```python
from build123d import *

# Parameters (mm, degrees)
SKETCH_1_R          = 5
EXTRUDE_4_DEPTH     = 12
FILLET_1_R          = 0.6
FILLET_2_R          = 0.6
EXTRUDE_5_DEPTH     = 6
SKETCH_3_R          = 2.55
CUT_EXTRUDE_1_DEPTH = 6
CHAMFER_1_SIZE      = 0.5
CHAMFER_4_SIZE      = 0.5
FILLET_4_R          = 0.5
FILLET_5_R          = 0.5
SKETCH_4_W          = 6.329239392
SKETCH_4_H          = 8
EXTRUDE_6_DEPTH     = 3.5
SKETCH_5_R          = 1.2
CUT_EXTRUDE_2_DEPTH = 3.5
FILLET_7_R          = 0.5


with BuildPart() as part:
    # ｽｹｯﾁ1 → ﾎﾞｽ - 押し出し4 (new body)
    with BuildSketch(Plane(origin=(0, 0, 0), x_dir=(1, 0, 0), z_dir=(0, 1, 0))):
        with Locations(Location((0, 0, 0), (0, 0, 270))):
            Circle(SKETCH_1_R)
        Polygon((-2.5, -0.925), (-2.5, 0.925), (-0.925, 0.925), (-0.925, 2.5), (0.925, 2.5), (0.925, 0.925), (2.5, 0.925), (2.5, -0.925), (0.925, -0.925), (0.925, -2.5), (-0.925, -2.5), (-0.925, -0.925), align=None, mode=Mode.SUBTRACT)
    extrude(amount=EXTRUDE_4_DEPTH)

    # ﾌｨﾚｯﾄ1
    fillet_1_edges = [part.edges().sort_by_distance(p)[0] for p in [
        (0.925, 6, -0.925),
    ]]
    fillet(fillet_1_edges, radius=FILLET_1_R)

    # ﾌｨﾚｯﾄ2
    fillet_2_edges = [part.edges().sort_by_distance(p)[0] for p in [
        (-0.925, 6, -0.925),
        (-0.925, 6, 0.925),
        (0.925, 6, 0.925),
    ]]
    fillet(fillet_2_edges, radius=FILLET_2_R)

    # ｽｹｯﾁ2 → ﾎﾞｽ - 押し出し5 (add)
    with BuildSketch(Plane.XZ):
        Polygon((6.92820323, 0), (3.464101615, 6), (-3.464101615, 6), (-6.92820323, 0), (-3.464101615, -6), (3.464101615, -6), align=None)
    extrude(amount=EXTRUDE_5_DEPTH)

    # ｽｹｯﾁ3 → ｶｯﾄ - 押し出し1 (cut)
    with BuildSketch(Plane.XZ.offset(6)):
        with Locations(Location((0, 0, 0), (0, 0, 270))):
            Circle(SKETCH_3_R)
    extrude(amount=-CUT_EXTRUDE_1_DEPTH, mode=Mode.SUBTRACT)

    # 面取り1
    chamfer_1_edges = [part.edges().sort_by_distance(p)[0] for p in [
        (0, -6, 2.55),
        (5.196152423, -6, -3),
        (5.196152423, -6, 3),
        (0, -6, 6),
        (-5.196152423, -6, 3),
        (-5.196152423, -6, -3),
        (0, -6, -6),
    ]]
    chamfer(chamfer_1_edges, length=CHAMFER_1_SIZE)

    # 面取り4
    chamfer_4_edges = [part.edges().sort_by_distance(p)[0] for p in [
        (2.5, 12, 0),
        (-2.0125, 12, -0.925),
        (-2.0125, 12, 0.925),
        (-2.5, 12, 0),
        (0, 12, -5),
        (2.0125, 12, -0.925),
        (1.100735931, 12, -1.100735931),
        (-0.925, 12, 2.0125),
        (2.0125, 12, 0.925),
        (0.925, 12, 2.0125),
        (1.100735931, 12, 1.100735931),
        (-1.100735931, 12, -1.100735931),
        (-1.100735931, 12, 1.100735931),
        (0.925, 12, -2.0125),
        (0, 12, -2.5),
        (0, 12, 2.5),
        (-0.925, 12, -2.0125),
    ]]
    chamfer(chamfer_4_edges, length=CHAMFER_4_SIZE)

    # ﾌｨﾚｯﾄ4
    fillet_4_edges = [part.edges().sort_by_distance(p)[0] for p in [
        (-3.464101615, -2.75, 6),
    ]]
    fillet(fillet_4_edges, radius=FILLET_4_R)

    # ﾌｨﾚｯﾄ5
    fillet_5_edges = [part.edges().sort_by_distance(p)[0] for p in [
        (3.464101615, -2.75, -6),
        (-3.464101615, -2.75, -6),
        (-6.92820323, -2.75, 0),
        (3.464101615, -2.75, 6),
        (6.92820323, -2.75, 0),
    ]]
    fillet(fillet_5_edges, radius=FILLET_5_R)

    # ｽｹｯﾁ4 → ﾎﾞｽ - 押し出し6 (add)
    with BuildSketch(Plane.XY.offset(-2.5)):
        with Locations((0.010806785, 4)):
            Rectangle(SKETCH_4_W, SKETCH_4_H)
    extrude(amount=-EXTRUDE_6_DEPTH)

    # ｽｹｯﾁ5 → ｶｯﾄ - 押し出し2 (cut)
    with BuildSketch(Plane(origin=(0, 0, -6), x_dir=(-1, 0, 0), z_dir=(0, 0, -1))):
        with Locations((0, 5)):
            Circle(SKETCH_5_R)
    extrude(amount=-CUT_EXTRUDE_2_DEPTH, mode=Mode.SUBTRACT)

    # ﾌｨﾚｯﾄ7
    fillet_7_edges = [part.edges().sort_by_distance(p)[0] for p in [
        (-4.7116556, 0, 1.673410144),
    ]]
    fillet(fillet_7_edges, radius=FILLET_7_R)


solid = part.part
```
Can you work these out from the model? Positions are in its coordinate system, mm. A direction names the side the tool comes from. Coordinates: 2 decimals unless noted, no trailing zeros. Loops run counter-clockwise (first coordinate to the right, second up) from the corner with the lowest first, then second, coordinate; pieces in that order, holes last.
1) For pin 1 (0.6 mm diameter, centred on y = 4, z = -5, fed in from -X); pin 2 (0.7 mm diameter, centred on x = -1.5, z = -1.5, fed in from -Y); pin 3 (0.5 mm diameter, centred on y = 7, z = 2, fed in from -X), each with a flat end and sliding along its axis, tell me the tip position at first contact or that it passes through.
2) Imagine slicing it at A-A on y = -4.5. List the corners of the cut face in (x, z) for me, plus the area to 3 significant figures.
3) Imagine slicing it at B-B on x = 0. State how many separate pieces and enclosed holes the cut face has, plus the area to 3 significant figures.
4) Which directions (+Z, -Z, +X, -X, +Y, -Y) give clear straight access to the entire face, cutting with the end or side of a thin tool? Please do faces 1 (the flat face through (0, -3, 6)), 2 (the flat face through (-3.154, 4, -5)), 3 (the flat face through (-1.5, 0, 1.5)), 4 (the flat face through (0, 1, -6)), 5 (the flat face through (0, 9, -2.5)).
5) Imagine slicing it at C-C on y = 5. List the corners of the cut face in (x, z) for me (3 decimals).
6) Imagine slicing it at D-D on x = 6. List the corners of the cut face in (y, z) for me, plus the area to 3 significant figures.
7) I need wall thicknesses on probe 1 along X at (y, z) = (-2.1, 0); probe 2 along X at (y, z) = (9, 2) (3 decimals); probe 3 along Z at (x, y) = (1, 11). Which ranges of each line are inside material? Lowest first, please.
8) Thinking about a two-plate mould opening in X: for faces 6 (the flat face through (0, 8, -5.4)), 7 (the flat face through (5.174, -2.712, -3.038)), 8 (the flat face through (0.925, 6, 2)), which applies, pulls with the +X half, pulls with the -X half, needs draft (parallel to the pull), parting line crosses it, or undercut?
Completed:
1. pin 1: stops at x = -3.15
1. pin 2: stops at y = 0
1. pin 3: stops at x = -4.68
2. outline: (-6.78, -0.25) - (-3.61, -5.75) arc R0.5 ccw to (-3.18, -6) - (3.18, -6) arc R0.5 ccw to (3.61, -5.75) - (6.78, -0.25) arc R0.5 ccw to (6.78, 0.25) - (3.61, 5.75) arc R0.5 ccw to (3.18, 6) - (-3.18, 6) arc R0.5 ccw to (-3.61, 5.75) - (-6.78, 0.25) arc R0.5 ccw to start; hole circle Ø5.1 at (0, 0)
2. area: 104 mm2
3. separate pieces: 3
3. enclosed holes: 0
3. area: 100 mm2
4. face 1: +Z, +X, -X, +Y, -Y
4. face 2: -Z, -X, +Y
4. face 3: -Y
4. face 4: -Z, +X, -X, +Y, -Y
4. face 5: +Y
5. outline: (-3.154, -6) - (-1.2, -6) - (-1.2, -2.5) - (-0.925, -2.5) - (-0.925, -1.525) arc R0.6 ccw to (-1.525, -0.925) - (-2.5, -0.925) - (-2.5, 0.925) - (-1.525, 0.925) arc R0.6 ccw to (-0.925, 1.525) - (-0.925, 2.5) - (0.925, 2.5) - (0.925, 1.525) arc R0.6 ccw to (1.525, 0.925) - (2.5, 0.925) - (2.5, -0.925) - (1.525, -0.925) arc R0.6 ccw to (0.925, -1.525) - (0.925, -2.5) - (1.2, -2.5) - (1.2, -6) - (3.175, -6) - (3.175, -3.862) arc R5 ccw (long way) to (-3.154, -3.88) - close
6. outline: (-6, -0.61) - (-5.5, -1.61) - (0, -1.61) - (0, 1.61) - (-5.5, 1.61) - (-6, 0.61) - close
6. area: 18.8 mm2
7. probe 1: x = -6.85 to -2.55, 2.55 to 6.85
7. probe 2: x = -4.583 to -0.925, 0.925 to 4.583
7. probe 3: z = -4.9 to -1.23, 1.23 to 4.9
8. face 6: needs draft
8. face 7: pulls with the +X half
8. face 8: undercut
